Work out the finished part from the listing and answer in its coordinate system (mm). Face numbers are marked on the shaded views. A direction names the side the tool comes from. Give positions to 0.01 mm unless a question says otherwise; leave off trailing zeros. Order: outer loops, then holes, each group sorted by start corner. A loop starts at its lowest first (then second) coordinate and runs counter-clockwise, first axis right, second up. Notation, with made-up numbers: M 49,3 L 71,3 A31 ccw 71,29 Z; hole C 74,-12 d11. An arc over 180 degrees is marked long. One line per item, written item: value.
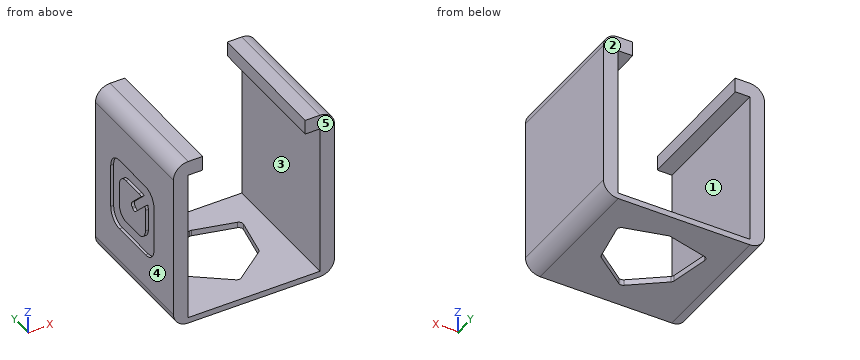
from build123d import *

# Parameters (mm, degrees)
F0_W      = 45
F0_H      = 45
F1_DEPTH  = 2
F2_DEPTH  = 5
F3_DEPTH  = 5
F4_W      = 5
F4_H      = 45
F5_DEPTH  = 57
F7_W      = 45
F7_H      = 5
F8_DEPTH  = 5
F6_W      = 45
F6_H      = 5
F9_DEPTH  = 5
F10_R     = 5
F12_DEPTH = 1


with BuildPart() as f1:
    # F0 (on Top) → F1 (new body)
    with BuildSketch(Plane.XY):
        with Locations((0, 4.82134892)):
            Rectangle(F0_W, F0_H)
        with BuildLine():
            ThreePointArc((-15.0511533834, 13.8031822317), (-14.8481410429, 14.8973282595), (-13.9471820002, 15.5505069059))
            Line((-13.9471820002, 15.5505069059), (-0.3671439173, 18.9786667044))
            ThreePointArc((-0.3671439173, 18.9786667044), (0, 19.0242921501), (0.3671439173, 18.9786667044))
            Line((0.3671439173, 18.9786667044), (13.9471820002, 15.5505069059))
            ThreePointArc((13.9471820002, 15.5505069059), (14.8481410429, 14.8973282595), (15.0511533834, 13.8031822317))
            Line((15.0511533834, 13.8031822317), (12.4127807629, 0.5539972479))
            ThreePointArc((12.4127807629, 0.5539972479), (12.2151536655, 0.0543391438), (11.854115567, -0.3436133433))
            Line((11.854115567, -0.3436133433), (0.9124501045, -8.7293459665))
            ThreePointArc((0.9124501045, -8.7293459665), (0, -9.0387852554), (-0.9124501045, -8.7293459665))
            Line((-0.9124501045, -8.7293459665), (-11.854115567, -0.3436133433))
            ThreePointArc((-11.854115567, -0.3436133433), (-12.2151536655, 0.0543391438), (-12.4127807629, 0.5539972479))
            Line((-12.4127807629, 0.5539972479), (-15.0511533834, 13.8031822317))
        make_face(mode=Mode.SUBTRACT)
    extrude(amount=F1_DEPTH)

    # F2 (add): a face of the model
    f2_faces = [f1.faces().sort_by_distance(p)[0] for p in [
        (-22.5, 4.82134892, 1),
    ]]
    extrude(f2_faces, amount=F2_DEPTH)

    # F3 (add): a face of the model
    f3_faces = [f1.faces().sort_by_distance(p)[0] for p in [
        (22.5, 4.82134892, 1),
    ]]
    extrude(f3_faces, amount=F3_DEPTH)

    # F4 (on face) → F5 (join)
    with BuildSketch(Plane.XY.offset(2)):
        with Locations((-25, 4.82134892)):
            Rectangle(F4_W, F4_H)
        with Locations((25, 4.82134892)):
            Rectangle(F4_W, F4_H)
    extrude(amount=F5_DEPTH)

    # F7 (on face) → F8 (join)
    with BuildSketch(Plane(origin=(22.5, 0, 0), x_dir=(0, -1, 0), z_dir=(-1, 0, 0))):
        with Locations((-4.82134892, 56.5)):
            Rectangle(F7_W, F7_H)
    extrude(amount=F8_DEPTH)

    # F6 (on face) → F9 (join)
    with BuildSketch(Plane.YZ.offset(-22.5)):
        with Locations((4.82134892, 56.5)):
            Rectangle(F6_W, F6_H)
    extrude(amount=F9_DEPTH)

    # F10
    f10_edges = [f1.edges().sort_by_distance(p)[0] for p in [
        (27.5, 4.821349, 0),
        (-27.5, 4.821349, 0),
        (-27.5, 4.821349, 59),
        (27.5, 4.821349, 59),
    ]]
    fillet(f10_edges, radius=F10_R)

    # F11 (on face) → F12 (cut)
    with BuildSketch(Plane(origin=(-27.5, 0, 0), x_dir=(0, -1, 0), z_dir=(-1, 0, 0))):
        with BuildLine():
            ThreePointArc((1.4999996684, 16.5000007302), (5.0355335744, 17.9644668242), (6.4999996684, 21.5000007302))
            Line((6.4999996684, 21.5000007302), (6.4999996684, 36.5000007302))
            ThreePointArc((6.4999996684, 36.5000007302), (5.0355335744, 40.0355346361), (1.4999996684, 41.5000007302))
            Line((1.4999996684, 41.5000007302), (-13.5000003316, 41.5000007302))
            ThreePointArc((-13.5000003316, 41.5000007302), (-17.0355342375, 40.0355346361), (-18.5000003316, 36.5000007302))
            Line((-18.5000003316, 36.5000007302), (-18.5000003316, 21.5000007302))
            ThreePointArc((-18.5000003316, 21.5000007302), (-17.0355342375, 17.9644668242), (-13.5000003316, 16.5000007302))
            Line((-13.5000003316, 16.5000007302), (1.4999996684, 16.5000007302))
        make_face()
        with BuildLine():
            Line((1.4999996684, 32.7500007302), (1.4999996684, 25.2500007302))
            ThreePointArc((1.4999996684, 25.2500007302), (0.4016500979, 22.5983503007), (-2.2500003316, 21.5000007302))
            Line((-2.2500003316, 21.5000007302), (-9.7500003316, 21.5000007302))
            ThreePointArc((-9.7500003316, 21.5000007302), (-12.401650761, 22.5983503007), (-13.5000003316, 25.2500007302))
            Line((-13.5000003316, 25.2500007302), (-13.5000003316, 32.7500007302))
            ThreePointArc((-13.5000003316, 32.7500007302), (-12.401650761, 35.4016511596), (-9.7500003316, 36.5000007302))
            Line((-9.7500003316, 36.5000007302), (-2.2500003316, 36.5000007302))
            ThreePointArc((-2.2500003316, 36.5000007302), (-1.5530488983, 36.4346660745), (-0.8803828421, 36.2409387033))
            Line((-0.8803828316, 36.2409387302), (-6.1767770816, 30.9445444802))
            ThreePointArc((-6.176777058, 30.9445444566), (-6.5428935816, 30.0606609802), (-6.176777058, 29.1767775037))
            Line((-6.1767770816, 29.1767774802), (-6.0000003316, 29.0000007302))
            Line((-6.0000003316, 29.0000007302), (-5.8232235816, 28.8232239802))
            ThreePointArc((-5.823223558, 28.8232240037), (-4.9393400816, 28.4571074802), (-4.0554566051, 28.8232240037))
            Line((-4.0554565816, 28.8232239802), (1.2409376684, 34.1196182302))
            ThreePointArc((1.2409376416, 34.1196182196), (1.4346650128, 33.4469521634), (1.4999996684, 32.7500007302))
        make_face(mode=Mode.SUBTRACT)
    extrude(amount=-F12_DEPTH, mode=Mode.SUBTRACT)


solid = f1.part
(1) Determine the mould class of the marked faces 3, 4 and 5 for opening direction X: pulls with the +X half, pulls with the -X half, needs draft (parallel to the pull), parting line crosses it, or undercut.
Findings:
face 3: undercut
face 4: pulls with the -X half
face 5: needs draft
(2) Section D-D, the plane z = 9.5 is taken. Give the vertices of the cut face in (x, y).
Findings:
outline: M -27.5,-17.68 L -22.5,-17.68 L -22.5,27.32 L -27.5,27.32 Z; M 22.5,-17.68 L 27.5,-17.68 L 27.5,27.32 L 22.5,27.32 Z
(3) Which of the six approach directions +Z, -Z, +X, -X, +Y, -Y give full straight-line access (tool end or side, diameter ignored) to the marked faces 1 and 2?
Findings:
face 1: +Y, -Y
face 2: +Z, -Z, +X, -X, +Y
(4) Find the intervals of material crossed by probe 1 along Z at (x, y) = (-21.5, 10); probe 2 along X at (y, z) = (25, 21); probe 3 along X at (y, z) = (15, 25), in increasing order. Write a range as from..to.
Findings:
probe 1: z = 0..2, 54..59
probe 2: x = -27.5..-22.5, 22.5..27.5
probe 3: x = -26.5..-22.5, 22.5..27.5
(5) Section B-B, the plane x = -19 is taken. Give the vertices of the cut face in (y, z), then the cut area to 3 significant figures.
Findings:
outline: M -17.68,0 L 27.32,0 L 27.32,2 L -17.68,2 Z; M -17.68,54 L 27.32,54 L 27.32,59 L -17.68,59 Z
area: 315 mm^2
(6) Section A-A, the plane z = 26.5 is taken. Give the vertices of the cut face in (x, y), then the cut area to 3 significant figures.
Findings:
outline: M -27.5,-17.68 L -22.5,-17.68 L -22.5,27.32 L -27.5,27.32 L -27.5,18.5 L -26.5,18.5 L -26.5,13.5 L -27.5,13.5 L -27.5,-1.5 L -26.5,-1.5 L -26.5,-6.5 L -27.5,-6.5 Z; M 22.5,-17.68 L 27.5,-17.68 L 27.5,27.32 L 22.5,27.32 Z
area: 440 mm^2
(7) Given P1, Ø0.5, axis at x = -27, y = 5.5, coming from the -Z side; P2, Ø2.5, axis at y = 5.5, z = 57, coming from the -X side; P3, Ø0.8, axis at x = -27, y = 2.5, coming from the +Z side, each flat-ended and moving along its own axis, determine where each tip first touches the part or whether it passes through.
Findings:
P1: stops at z = 2.37
P2: stops at x = -27.18
P3: stops at z = 56.86
